Here's how the part is built. I have some questions about the finished solid (model axes, mm). A direction names the side the tool comes from. Round coordinates to 2 decimals unless told otherwise and drop trailing zeros. Write each loop counter-clockwise with the first axis right and the second up, starting at its lowest first coordinate (ties: lowest second). Pieces come first, ordered by that corner, then holes. Notation, with made-up numbers: (53, 28.25) -> (97, 28.25) arc R20 ccw to (97, 35.25) -> close; hole circle Ø10 at (51, 37). An arc over 180 degrees is marked (long way). Answer in a Markdown table with one row per item. Add a question column.
from build123d import *

# Parameters (mm, degrees)
F0_R      = 7.5
F1_DEPTH  = 40
F3_DEPTH  = 2.5
F4_R      = 2
F5_R      = 2.25
F6_DEPTH  = 2.5
F7_W      = 6
F7_H      = 20
F7_R      = 2.25
F8_DEPTH  = 2.5
F9_R      = 2
F11_DEPTH = 40


with BuildPart() as f1:
    # F0 (on Front) → F1 (new body)
    with BuildSketch(Plane.XZ):
        Circle(F0_R)
    extrude(amount=F1_DEPTH)

    # F2 (on face) → F3 (join)
    with BuildSketch(Plane(origin=(0, 0, 0), x_dir=(-1, 0, 0), z_dir=(0, 1, 0))):
        with BuildLine():
            Line((3, 20), (-3, 20))
            Line((-3, 20), (-3, 6.873864))
            ThreePointArc((-3, 6.873864), (0, 7.5), (3, 6.873864))
            Line((3, 6.873864), (3, 20))
        make_face()
        with BuildLine():
            ThreePointArc((3, 6.873864), (0, 7.5), (-3, 6.873864))
            Line((-3, 6.873864), (-3, 0))
            Line((-3, 0), (3, 0))
            Line((3, 0), (3, 6.873864))
        make_face()
    extrude(amount=F3_DEPTH)

    # F4
    f4_edges = [f1.edges().sort_by_distance(p)[0] for p in [
        (3, 1.25, 20),
        (-3, 1.25, 20),
        (3, 1.25, 0),
        (-3, 1.25, 0),
    ]]
    fillet(f4_edges, radius=F4_R)

    # F5 (on face) → F6 (join)
    with BuildSketch(Plane(origin=(0, 2.5, 0), x_dir=(-1, 0, 0), z_dir=(0, 1, 0))):
        with Locations((0, 15.968132)):
            Circle(F5_R)
    extrude(amount=F6_DEPTH)

    # F7 (on face) → F8 (join)
    with BuildSketch(Plane(origin=(0, 5, 0), x_dir=(-1, 0, 0), z_dir=(0, 1, 0))):
        with Locations((0, 10)):
            Rectangle(F7_W, F7_H)
        with Locations((0, 15.968132)):
            Circle(F7_R, mode=Mode.SUBTRACT)
        with Locations((0, 15.968132)):
            Circle(F7_R)
    extrude(amount=F8_DEPTH)

    # F9
    f9_edges = [f1.edges().sort_by_distance(p)[0] for p in [
        (3, 6.25, 20),
        (-3, 6.25, 20),
        (3, 6.25, 0),
        (-3, 6.25, 0),
    ]]
    fillet(f9_edges, radius=F9_R)

    # F10 (on face) → F11 (join)
    with BuildSketch(Plane(origin=(0, 7.5, 0), x_dir=(-1, 0, 0), z_dir=(0, 1, 0))):
        with BuildLine():
            Line((3, 2), (3, 6.873864))
            ThreePointArc((3, 6.873864), (0, 7.5), (-3, 6.873864))
            Line((-3, 6.873864), (-3, 2))
            ThreePointArc((-3, 2), (-2.414214, 0.585786), (-1, 0))
            Line((-1, 0), (1, 0))
            ThreePointArc((1, 0), (2.414214, 0.585786), (3, 2))
        make_face()
        with BuildLine():
            ThreePointArc((-3, 6.873864), (-4.107919, -6.27495), (7.5, 0))
            ThreePointArc((7.5, 0), (6.27495, 4.107919), (3, 6.873864))
            Line((3, 6.873864), (3, 2))
            ThreePointArc((3, 2), (2.414214, 0.585786), (1, 0))
            Line((1, 0), (-1, 0))
            ThreePointArc((-1, 0), (-2.414214, 0.585786), (-3, 2))
            Line((-3, 2), (-3, 6.873864))
        make_face()
    extrude(amount=F11_DEPTH)


solid = f1.part
Item 1: If we section it at C-C on x = 0: Please give me the cut outline in (y, z), then the cut area to 3 significant figures.
Item 2: If we section it at D-D on y = -29: Please give me the cut outline in (x, z).
Item 3: I need wall thicknesses on line 1 along Y through (x, z) = (4, 0.25); line 2 along Y through (x, z) = (-2.5, 1); line 3 along X through (y, z) = (-33, 0.25). Which ranges of each line are inside material? Lowest first, please. Write a range as from..to.
Item 4: If we section it at A-A on z = 12.75: Please give me the cut outline in (x, y).
Item 5: On a 3-axis mill with a long thin cutter (end or side, diameter ignored), from which of +Z, -Z, +X, -X, +Y, -Y can I reach the whole of each face in a straight line? I mean faces 5 (the cylindrical face through (-2.4, 6.27, 0.57)), 6 (the flat face through (-3, 6, 10)), 7 (the cylindrical face through (0.3, 3.7, 18.2)), 8 (the flat face through (3, 6, 10)). Say none if no direction works.
Item 6: If we mould it in two halves opening along Y, with no side actions, what happens to faces 1 (the flat face through (0, 7.5, 14)), 2 (the cylindrical face through (-2.43, 1.27, 0.6)), 3 (the flat face through (0, -40, 0)), 4 (the cylindrical face through (-7.493, -19.72, 0.33))? For each: pulls with the +Y half, pulls with the -Y half, needs draft (parallel to the pull), parting line crosses it, or undercut.
Item 7: If we section it at B-B on x = 5: Please give me the cut outline in (y, z), then the cut area to 3 significant figures.
Item 8: For P1, Ø2, axis at y = 6.5, z = 9, coming from the -X side; P2, Ø6.5, axis at x = -1.5, z = 12.5, coming from the +Y side; P3, Ø10, axis at y = 25.5, z = 6, coming from the -X side; P4, Ø8, axis at x = -3.5, z = 7, coming from the -Y side, each with a flat end and sliding along its axis, tell me the tip position at first contact or that it passes through.
Results list:
| question | item | result |
|---|---|---|
| 1 | outline | (-40, -7.5) -> (0, -7.5) -> (0, 0) -> (2.5, 0) -> (2.5, 13.72) -> (5, 13.72) -> (5, 0) -> (7.5, 0) -> (7.5, -7.5) -> (47.5, -7.5) -> (47.5, 7.5) -> (7.5, 7.5) -> (7.5, 20) -> (5, 20) -> (5, 18.22) -> (2.5, 18.22) -> (2.5, 20) -> (0, 20) -> (0, 7.5) -> (-40, 7.5) -> close |
| 1 | area | 1,310 mm² |
| 2 | outline | circle Ø15 at (0, 0) |
| 3 | line 1 | -40..0, 7.5..47.5 |
| 3 | line 2 | -40..2.5, 5..47.5 |
| 3 | line 3 | -7.5..7.5 |
| 4 | outline | (-3, 0) -> (3, 0) -> (3, 2.5) -> (-3, 2.5) -> close; (-3, 5) -> (3, 5) -> (3, 7.5) -> (-3, 7.5) -> close |
| 5 | face 5 | -Z, -X |
| 5 | face 6 | +Z, -Z, -X |
| 5 | face 7 | none |
| 5 | face 8 | +Z, -Z, +X |
| 6 | face 1 | pulls with the +Y half |
| 6 | face 2 | undercut |
| 6 | face 3 | pulls with the -Y half |
| 6 | face 4 | needs draft |
| 7 | outline | (-40, -5.59) -> (0, -5.59) -> (0, 5.59) -> (-40, 5.59) -> close; (7.5, -5.59) -> (47.5, -5.59) -> (47.5, 5.59) -> (7.5, 5.59) -> close |
| 7 | area | 894 mm² |
| 8 | P1 | x = -3 |
| 8 | P2 | y = 7.5 |
| 8 | P3 | x = -7.43 |
| 8 | P4 | y = -40 |
